Geometry check sheet. Reference: the model listing, model coordinates, mm. Face numbers are marked on the shaded views. Give positions to 0.01 mm unless a question says otherwise; leave off trailing zeros.
1. Go/stop test with flat-tipped pins: pin 1 Ø5 at (y, z) = (-2.5, 21) entering from -X; pin 2 Ø2.5 at (x, y) = (-5.5, 0) entering from +Z; pin 3 Ø2 at (y, z) = (-15.5, 7) entering from +X. Record where each tip stops, or that it passes through.
2. Material ranges on L1, parallel to X at y = 5, z = 17.25; L2, parallel to X at y = 0, z = 21.75; L3, parallel to X at y = -4.5, z = 13.5, recorded low to high.
3. Release check for a two-part mould opening along X. For the marked faces 1, 2 and 3 record: +X half, -X half, draft (parallel to the pull), parting line (faces both ways), or undercut.
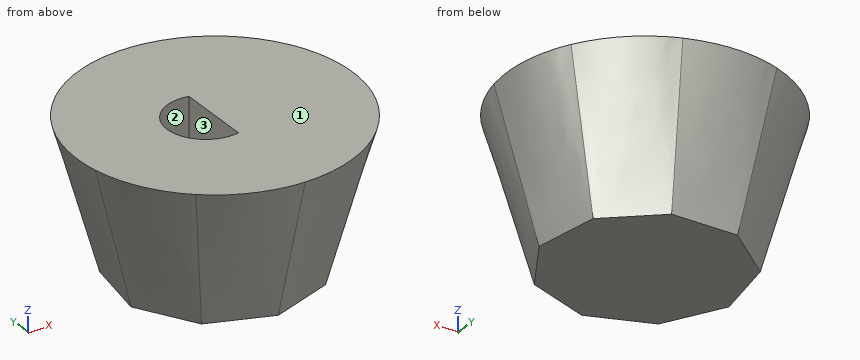
from build123d import *

# Parameters (mm, degrees)
F5_DEPTH = 10.414


# Not quite as in the source:
# - the arcs of a loft's sections are written as splines that run evenly, so that the points pair up as in the source's solid


with BuildPart() as f3:
    # F0 (on Top) → F3 section 0
    with BuildSketch(Plane.XY):
        Polygon((10.7835912141, -12.8513835704), (16.5214202528, -2.9131721502), (14.5286931401, 8.3881448954), (5.7378290387, 15.7645557206), (-5.7378290387, 15.7645557206), (-14.5286931401, 8.3881448954), (-16.5214202528, -2.9131721502), (-10.7835912141, -12.8513835704), (0, -16.7762897909), align=None)
    # F2 (on offset) → F3 section 1
    with BuildSketch(Plane.XY.offset(25.4)):
        with BuildLine():
            add(Edge.make_bspline(
                [(15.363307355, -18.3092767345), (17.4936884395, -16.5216747522), (19.3084205069, -14.3589612913), (22.0894355037, -9.5421020203), (23.0550342683, -6.8891412184), (23.5379524545, -4.1503760884)],
                knots=[0, 0, 0, 0, 0.5, 0.5, 1, 1, 1, 1], degree=3))
            add(Edge.make_bspline(
                [(23.5379524545, -4.1503760884), (24.0208706408, -1.4116109583), (24.0208706408, 1.4116109583), (23.0550342683, 6.8891412184), (22.0894355037, 9.5421020203), (20.6989280053, 11.9505316558)],
                knots=[0, 0, 0, 0, 0.5, 0.5, 1, 1, 1, 1], degree=3))
            add(Edge.make_bspline(
                [(20.6989280053, 11.9505316558), (19.3084205069, 14.3589612913), (17.4936884395, 16.5216747522), (13.2329262705, 20.0968787168), (10.7879443702, 21.5084896751), (8.1746450995, 22.4596528229)],
                knots=[0, 0, 0, 0, 0.5, 0.5, 1, 1, 1, 1], degree=3))
            add(Edge.make_bspline(
                [(8.1746450995, 22.4596528229), (5.5613458287, 23.4108159707), (2.7810149968, 23.9010633116), (-2.7810149968, 23.9010633116), (-5.5613458287, 23.4108159707), (-8.1746450995, 22.4596528229)],
                knots=[0, 0, 0, 0, 0.5, 0.5, 1, 1, 1, 1], degree=3))
            add(Edge.make_bspline(
                [(-8.1746450995, 22.4596528229), (-10.7879443702, 21.5084896751), (-13.2329262705, 20.0968787168), (-17.4936884395, 16.5216747522), (-19.3084205069, 14.3589612913), (-20.6989280053, 11.9505316558)],
                knots=[0, 0, 0, 0, 0.5, 0.5, 1, 1, 1, 1], degree=3))
            add(Edge.make_bspline(
                [(-20.6989280053, 11.9505316558), (-22.0894355037, 9.5421020203), (-23.0550342683, 6.8891412184), (-24.0208706408, 1.4116109583), (-24.0208706408, -1.4116109583), (-23.5379524545, -4.1503760884)],
                knots=[0, 0, 0, 0, 0.5, 0.5, 1, 1, 1, 1], degree=3))
            add(Edge.make_bspline(
                [(-23.5379524545, -4.1503760884), (-23.0550342683, -6.8891412184), (-22.0894355037, -9.5421020203), (-19.3084205069, -14.3589612913), (-17.4936884395, -16.5216747522), (-15.363307355, -18.3092767345)],
                knots=[0, 0, 0, 0, 0.5, 0.5, 1, 1, 1, 1], degree=3))
            add(Edge.make_bspline(
                [(-15.363307355, -18.3092767345), (-13.2329262705, -20.0968787168), (-10.7879443702, -21.5084896751), (-5.5613458287, -23.4108159707), (-2.7810149968, -23.9010633116), (0, -23.9010633116)],
                knots=[0, 0, 0, 0, 0.5, 0.5, 1, 1, 1, 1], degree=3))
            add(Edge.make_bspline(
                [(0, -23.9010633116), (2.7810149968, -23.9010633116), (5.5613458287, -23.4108159707), (10.7879443702, -21.5084896751), (13.2329262705, -20.0968787168), (15.363307355, -18.3092767345)],
                knots=[0, 0, 0, 0, 0.5, 0.5, 1, 1, 1, 1], degree=3))
        make_face()
    loft(ruled=True)

    # F4 (on face) → F5 (cut)
    with BuildSketch(Plane.XY.offset(25.4)):
        with BuildLine():
            Line((0, -6.2373387627), (0, 6.8825809285))
            ThreePointArc((0, 6.8825809285), (-8.1053000761, 0.3226210829), (0, -6.2373387627))
        make_face()
    extrude(amount=-F5_DEPTH, mode=Mode.SUBTRACT)


solid = f3.part
Result:
1. pin 1: stops at x = -23.23
1. pin 2: stops at z = 14.99
1. pin 3: stops at x = 11.85
2. L1: x = -20.71 to -6.21, 0 to 20.71
2. L2: x = -22.77 to -8.1, 0 to 22.77
2. L3: x = -19.94 to 19.94
3. face 1: draft
3. face 2: undercut
3. face 3: undercut
